Build history of the part. All positions in model axes, mm. A direction names the side the tool comes from. Coordinates: 2 decimals unless noted, no trailing zeros. Loops run counter-clockwise (first coordinate to the right, second up) from the corner with the lowest first, then second, coordinate; pieces in that order, holes last. Notation, with made-up numbers: (-7, 45.25) -> (37, 45.25) arc R28 cw to (37, 73.25) -> close; hole circle Ø4 at (41, -35). An arc over 180 degrees is marked (long way). One line per item, written item: value. Start each with the question number.
```python
from build123d import *

# Parameters (mm, degrees)
SKETCH_1_W          = 60
SKETCH_1_H          = 30
EXTRUDE_1_DEPTH     = 1
CUT_EXTRUDE_1_REACH = 44.438
SKETCH_2_R          = 1.6
SKETCH_2_3_R        = 1.6
CUT_EXTRUDE_2_DEPTH = 1
SKETCH_3_W          = 11.33901572
SKETCH_3_H          = 5.18636438
EXTRUDE_2_DEPTH     = 20
SKETCH_5_W          = 3.694083694
SKETCH_5_H          = 6.454031282
SKETCH_5_W_2        = 3.311937105
SKETCH_5_H_2        = 6.538952746
SKETCH_5_W_3        = 4.308869274
SKETCH_5_H_3        = 7.904993255
EXTRUDE_3_DEPTH     = 5


with BuildPart() as part:
    # 草图1 → 凸台-拉伸1 (new body)
    with BuildSketch(Plane.XY):
        with Locations((0, 15)):
            Rectangle(SKETCH_1_W, SKETCH_1_H)
    extrude(amount=EXTRUDE_1_DEPTH)

    # 草图2 → 切除-拉伸1 (cut, up to next)
    with BuildSketch(Plane.XY.offset(1), mode=Mode.PRIVATE) as cut_extrude_1_sk1:
        with Locations((-26.155810983, 4.958036855)):
            Circle(SKETCH_2_R)
    cut_extrude_1_tool1 = extrude(cut_extrude_1_sk1.sketch, amount=-CUT_EXTRUDE_1_REACH, mode=Mode.PRIVATE) & part.part
    add(cut_extrude_1_tool1.solids().sort_by_distance((-26.155811, 4.958037, 1))[0], mode=Mode.SUBTRACT)

    # 草图2<3> → 切除-拉伸2 (cut)
    with BuildSketch(Plane.XY.offset(1)):
        with Locations((-26.155810983, 26.782853162)):
            Circle(SKETCH_2_3_R)
        with Locations((-26.155810983, 4.958036855)):
            Circle(SKETCH_2_3_R)
        with Locations((24.712146091, 26.782853162)):
            Circle(SKETCH_2_3_R)
        with Locations((24.712146091, 4.958036855)):
            Circle(SKETCH_2_3_R)
    extrude(amount=-CUT_EXTRUDE_2_DEPTH, mode=Mode.SUBTRACT)

    # 草图3 → 凸台-拉伸2 (add)
    with BuildSketch(Plane.XY.offset(1)):
        with Locations((-1.41614663, 24.527155888)):
            Rectangle(SKETCH_3_W, SKETCH_3_H)
    extrude(amount=EXTRUDE_2_DEPTH)

    # 草图5 → 凸台-拉伸3 (add)
    with BuildSketch(Plane.XY):
        with Locations((-25.115523047, 19.352225042)):
            Rectangle(SKETCH_5_W, SKETCH_5_H)
        with Locations((-25.311844501, 11.600994733)):
            Rectangle(SKETCH_5_W_2, SKETCH_5_H_2)
        with Locations((24.643382961, 16.097003055)):
            Rectangle(SKETCH_5_W_3, SKETCH_5_H_3)
    extrude(amount=EXTRUDE_3_DEPTH)


solid = part.part
```
Item 1: Band-saw the part on A-A, the plane x = -4. List the corners of the cut face in (y, z), and give its area (3 significant figures).
Item 2: Tool access for faces 5 (the face through (-25, 16.125, 3)), 6 (the face through (25, 12.145, 3)), 7 (the face through (26.798, 16, 3)): list every direction of +Z, -Z, +X, -X, +Y, -Y with a clear straight run to the whole face (end or side of a thin tool).
Item 3: Drop flat-ended pins along their axis: pin 1 Ø1.3 at (x, y) = (24.5, 17.5) entering from +Z; pin 2 Ø1.2 at (x, z) = (24.5, 4) entering from +Y; pin 3 Ø1.6 at (y, z) = (24, 15) entering from -X. Give the stop position or say it passes through.
Item 4: Probe probe 1 along X at (y, z) = (19.5, 4.25); probe 2 along X at (y, z) = (12.5, 2); probe 3 along Z at (x, y) = (0.5, 2.25). List the from-to ranges inside material, lowest first.
Item 5: Two-plate mould, pull along Y, no slides. Class faces 1 (the face through (-25.42, 25.36, 0.51)), 2 (the face through (25.45, 25.363, 0.507)), 3 (the face through (-7.086, 24, 11)), 4 (the face through (-25, 8.332, 3)): +Y half, -Y half, draft (parallel to the pull), parting line (faces both ways), or undercut.
Item 6: Band-saw the part on D-D, the plane z = 7.5. List the corners of the cut face in (x, y), and give its area (3 significant figures).
Item 7: Band-saw the part on B-B, the plane y = 9. List the corners of the cut face in (x, z).
Item 8: Band-saw the part on C-C, the plane y = 27.75. List the corners of the cut face in (x, z), and give its area (3 significant figures).
Worked out:
1. outline: (0, 0) -> (30, 0) -> (30, 1) -> (27.12, 1) -> (27.12, 21) -> (21.93, 21) -> (21.93, 1) -> (0, 1) -> close
1. area: 134 mm²
2. face 5: +Z, -X
2. face 6: +Z, +X, -Y
2. face 7: +Z, +X, +Y, -Y
3. pin 1: stops at z = 5
3. pin 2: stops at y = 20.05
3. pin 3: stops at x = -7.09
4. probe 1: x = -26.96 to -23.27, 22.49 to 26.8
4. probe 2: x = -26.97 to -23.66, 22.49 to 26.8
4. probe 3: z = 0 to 1
5. face 1: undercut
5. face 2: undercut
5. face 3: draft
5. face 4: -Y half
6. outline: (-7.09, 21.93) -> (4.25, 21.93) -> (4.25, 27.12) -> (-7.09, 27.12) -> close
6. area: 58.8 mm²
7. outline: (-30, 0) -> (30, 0) -> (30, 1) -> (-23.66, 1) -> (-23.66, 5) -> (-26.97, 5) -> (-26.97, 1) -> (-30, 1) -> close
8. outline: (-30, 0) -> (-27.43, 0) -> (-27.43, 1) -> (-30, 1) -> close; (-24.88, 0) -> (23.44, 0) -> (23.44, 1) -> (-24.88, 1) -> close; (25.99, 0) -> (30, 0) -> (30, 1) -> (25.99, 1) -> close
8. area: 54.9 mm²
